For this review, take the finished solid that the model builds, in its own axes (mm). A direction names the side the tool comes from. Coordinates: 2 decimals unless noted, no trailing zeros. Write each loop counter-clockwise with the first axis right and the second up, starting at its lowest first coordinate (ties: lowest second). Pieces come first, ordered by that corner, then holes.
1) We need section A-A on z = 6.5. Write out the cut boundary in (x, y).
2) We need section B-B on y = -27. Write out the cut boundary in (x, z).
3) Insertion check: P1, Ø7.5, axis at x = -3, y = -37.5, coming from the -Z side; P2, Ø3, axis at y = -34.5, z = 12.5, coming from the +X side; P3, Ø7.5, axis at x = -11.5, z = 14, coming from the -Y side. Each pin has a flat end and moves straight along its axis. Give the tip position at first contact, or say it passes through.
4) For faces 1 (the face through (-8, -25.4, 13)), 2 (the face through (-25, -19, 0)), list the 3-axis set-ups (+Z, -Z, +X, -X, +Y, -Y) from which the entire face can be reached by the end or side of a thin tool; tool diameter is ignored.
5) To check wall thickness, follow line 1 along X through (y, z) = (-46, 12); line 2 along Z through (x, y) = (-1.5, -44.5); line 3 along Y through (x, z) = (-7.5, 9.5). State the ranges of each line that lie inside material, in increasing order.
from build123d import *

# Parameters (mm, degrees)
F0_W     = 50.8
F0_H     = 50.8
F1_DEPTH = 50.8
F2_W     = 25.4
F2_H     = 25.4
F3_DEPTH = 50.8
F4_W     = 25.4
F4_H     = 25.4
F5_DEPTH = 101.6
F6_W     = 26.5487587631
F6_H     = 25.4
F7_DEPTH = 25.4


with BuildPart() as f1:
    # F0 (on Front) → F1 (new body)
    with BuildSketch(Plane.XZ):
        with Locations((-19.4743440211, 25.4)):
            Rectangle(F0_W, F0_H)
    extrude(amount=F1_DEPTH)

    # F2 (on Top) → F3 (cut)
    with BuildSketch(Plane.XY):
        with Locations((-32.7472079873, -12.7)):
            Rectangle(F2_W, F2_H)
        with Locations((-32.7472079873, -38.1)):
            Rectangle(F2_W, F2_H)
        with Locations((-7.3472079873, -38.1)):
            Rectangle(F2_W, F2_H)
    extrude(amount=-F3_DEPTH, mode=Mode.SUBTRACT)

    # F4 (on Top) → F5 (cut)
    with BuildSketch(Plane.XY):
        with Locations((-12.7, -17.0889281064)):
            Rectangle(F4_W, F4_H)
    extrude(amount=-F5_DEPTH, mode=Mode.SUBTRACT)

    # F6 (on face) → F7 (cut)
    with BuildSketch(Plane.XZ.offset(50.8)):
        with Locations((-7.3487234026, 12.7)):
            Rectangle(F6_W, F6_H)
    extrude(amount=-F7_DEPTH, mode=Mode.SUBTRACT)


solid = f1.part
Result:
1. outline: (-44.87, -50.8) - (-20.62, -50.8) - (-20.62, -25.4) - (5.93, -25.4) - (5.93, 0) - (-44.87, 0) - close
2. outline: (-44.87, 0) - (-20.62, 0) - (-20.62, 25.4) - (5.93, 25.4) - (5.93, 50.8) - (-44.87, 50.8) - close
3. P1: stops at z = 25.4
3. P2: stops at x = -20.62
3. P3: stops at y = -25.4
4. face 1: -Z, +X, -Y
4. face 2: -Z, +X, -X, +Y, -Y
5. line 1: x = -44.87 to -20.62
5. line 2: z = 25.4 to 50.8
5. line 3: y = -25.4 to 0
